Geometry check sheet. Reference: the model listing, model coordinates, mm. Face numbers are marked on the shaded views. A direction names the side the tool comes from. Round coordinates to 2 decimals unless told otherwise and drop trailing zeros. Order: outer loops, then holes, each group sorted by start corner. A loop starts at its lowest first (then second) coordinate and runs counter-clockwise, first axis right, second up.
```python
from build123d import *

# Parameters (mm, degrees)
SALIENTE_EXTRUIR1_DEPTH = 4.5
CROQUIS3_R              = 2.9
CROQUIS3_R_2            = 1
CORTAR_EXTRUIR1_DEPTH   = 13.30662017
REDONDEO1_R             = 50
CORTAR_EXTRUIR2_START   = -2.25
CROQUIS9_R              = 1
CORTAR_EXTRUIR2_DEPTH   = 1
SALIENTE_EXTRUIR2_START = -0.6
CROQUIS7_R              = 2.9
CROQUIS7_R_2            = 1.5
SALIENTE_EXTRUIR2_DEPTH = 0.6


with BuildPart() as part:
    # Croquis1 → Saliente-Extruir1 (new body)
    with BuildSketch(Plane(origin=(0, 0, 0), x_dir=(1, 0, 0), z_dir=(0, 1, 0))):
        with BuildLine():
            Line((-3.9, 0), (-2.5, 8.27))
            ThreePointArc((-2.5, 8.27), (0, 10.77), (2.5, 8.27))
            Line((2.5, 8.27), (3.9, 0))
            ThreePointArc((3.9, 0), (0, -3.9), (-3.9, 0))
        make_face()
    extrude(amount=SALIENTE_EXTRUIR1_DEPTH)

    # Croquis3 → Cortar-Extruir1 (cut, through all)
    with BuildSketch(Plane(origin=(0, 4.5, 0), x_dir=(1, 0, 0), z_dir=(0, 1, 0))):
        with Locations(Location((0, 0, 0), (0, 0, 270))):
            Circle(CROQUIS3_R)
        with Locations(Location((0, 8.27, 0), (0, 0, 270))):
            Circle(CROQUIS3_R_2)
    extrude(amount=-CORTAR_EXTRUIR1_DEPTH, mode=Mode.SUBTRACT)

    # Redondeo1
    redondeo1_edges = [part.edges().sort_by_distance(p)[0] for p in [
        (-2.5, 2.25, -8.27),
        (2.5, 2.25, -8.27),
    ]]
    fillet(redondeo1_edges, radius=REDONDEO1_R)

    # Croquis9 → Cortar-Extruir2 (cut, symmetric)
    with BuildSketch(Plane(origin=(0, 4.5, 0), x_dir=(1, 0, 0), z_dir=(0, 1, 0)).offset(CORTAR_EXTRUIR2_START)):
        with BuildLine():
            Line((3.682695525, 1.283648577), (2.750594125, 6.789704705))
            ThreePointArc((2.750594125, 6.789704705), (2.606305638, 7.69206861), (2.478532652, 8.596918789))
            ThreePointArc((2.478532652, 8.596918789), (0, 10.77), (-2.478532652, 8.596918789))
            ThreePointArc((-2.478532652, 8.596918789), (-2.606305638, 7.69206861), (-2.750594125, 6.789704705))
            Line((-2.750594125, 6.789704705), (-3.682695525, 1.283648577))
            ThreePointArc((-3.682695525, 1.283648577), (0, 3.9), (3.682695525, 1.283648577))
        make_face()
        with Locations(Location((0, 8.27, 0), (0, 0, 270))):
            Circle(CROQUIS9_R, mode=Mode.SUBTRACT)
    extrude(amount=CORTAR_EXTRUIR2_DEPTH, both=True, mode=Mode.SUBTRACT)

    # Croquis7 → Saliente-Extruir2 (add)
    with BuildSketch(Plane.XZ.offset(SALIENTE_EXTRUIR2_START)):
        with Locations(Location((0, 0, 0), (0, 0, 90))):
            Circle(CROQUIS7_R)
        with Locations(Location((0, 0, 0), (0, 0, 270))):
            Circle(CROQUIS7_R_2, mode=Mode.SUBTRACT)
    extrude(amount=SALIENTE_EXTRUIR2_DEPTH)


solid = part.part
```
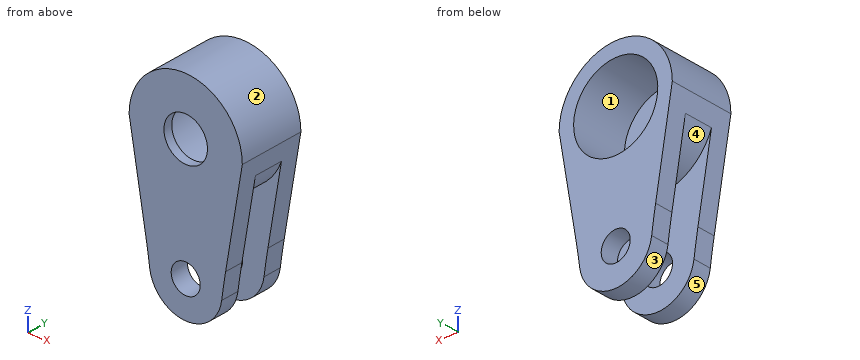
(1) Set-up check for the marked faces 4 and 5: record each of +Z, -Z, +X, -X, +Y, -Y from which the full face is reachable in a straight line by a thin tool's end or side.
Returned:
face 4: -Z
face 5: -Z, +Y, -Y
(2) Sectioned sample at D-D, the plane y = 2.95. Record the cut outline in (x, z).
Returned:
outline: (-3.9, 0) - (-3.68, -1.28) arc R3.9 ccw to (3.68, -1.28) - (3.9, 0) arc R3.9 ccw to start; hole circle Ø5.8 at (0, 0)
(3) Depth check by flat-ended pin: P1, Ø1, axis at x = -2, z = 1, coming from the +Y side; P2, Ø2, axis at x = 3, z = -9, coming from the -Y side; P3, Ø2, axis at x = 1.5, y = 3, coming from the +Z side; P4, Ø1.8, axis at x = 0, z = -8.27, coming from the +Y side. Enter the tip coordinate at first touch or a pass-through.
Returned:
P1: stops at y = 0.6
P2: stops at y = 0
P3: stops at z = 3.87
P4: passes through
(4) Material ranges on line 1 (Z direction, x = 0.75, y = 3.7); line 2 (Y direction, x = 1, z = -9.5); line 3 (X direction, y = 2.9, z = 1), recorded low to high.
Returned:
line 1: z = -10.65 to -8.93, -7.61 to -2.8, 2.8 to 3.83
line 2: y = 0 to 1.25, 3.25 to 4.5
line 3: x = -3.77 to -2.72, 2.72 to 3.77
(5) Sectioned sample at B-B, the plane z = 1. Record the cut outline in (x, y).
Returned:
outline: (-3.77, 0) - (-1.12, 0) - (-1.12, 0.6) - (-2.72, 0.6) - (-2.72, 4.5) - (-3.77, 4.5) - close; (1.12, 0) - (3.77, 0) - (3.77, 4.5) - (2.72, 4.5) - (2.72, 0.6) - (1.12, 0.6) - close
(6) Sectioned sample at C-C, the plane x = 0. Record the cut outline in (y, z).
Returned:
outline: (0, -10.77) - (1.25, -10.77) - (1.25, -9.27) - (0, -9.27) - close; (0, -7.27) - (1.25, -7.27) - (1.25, -3.9) - (3.25, -3.9) - (3.25, -7.27) - (4.5, -7.27) - (4.5, -2.9) - (0.6, -2.9) - (0.6, -1.5) - (0, -1.5) - close; (0, 1.5) - (0.6, 1.5) - (0.6, 2.9) - (4.5, 2.9) - (4.5, 3.9) - (0, 3.9) - close; (3.25, -10.77) - (4.5, -10.77) - (4.5, -9.27) - (3.25, -9.27) - close
(7) Sectioned sample at A-A, the plane y = 4.2. Record the cut outline in (x, z), and give its area (3 significant figures).
Returned:
outline: (-3.9, 0) - (-2.75, -6.79) arc R50 cw to (-2.48, -8.6) arc R2.5 ccw to (2.48, -8.6) arc R50 cw to (2.75, -6.79) - (3.9, 0) arc R3.9 ccw to start; hole circle Ø5.8 at (0, 0); hole circle Ø2 at (0, -8.27)
area: 57.1 mm2
(8) Draft check along Z on the marked faces 1, 2 and 3. Enter one of: released by +Z, released by -Z, zero draft, split by the parting line, or undercut.
Returned:
face 1: undercut
face 2: released by +Z
face 3: released by -Z
